from build123d import *

# Parameters (mm, degrees)
FILLET1_R   = 0.2
HEX_2_DEPTH = 1.56


with BuildPart() as part:
    # BodySke → BaseBody (revolve)
    with BuildSketch(Plane.XY):
        with BuildLine():
            Line((12.75, 0), (12.75, 2.055))
            Line((12.75, 2.055), (12.305, 2.5))
            Line((12.305, 2.5), (2.75, 2.5))
            Line((2.75, 2.5), (2.75, 4.75))
            Line((2.75, 4.75), (2.37, 4.75))
            ThreePointArc((2.37, 4.75), (0.992680215, 3.754414901), (0, 2.375))
            Line((0, 2.375), (0, 0))
            Line((0, 0), (12.75, 0))
        make_face()
    revolve(axis=Axis((0, 0, 0), (1, 0, 0)))

    # Fillet1
    fillet1_edges = [part.edges().sort_by_distance(p)[0] for p in [
        (2.75, -2.5, 0),
    ]]
    fillet(fillet1_edges, radius=FILLET1_R)

    # Sketch2 → PreBroach (revolve, cut)
    with BuildSketch(Plane.XY):
        Polygon((0, 1.5), (1.56, 1.5), (2.426025404, 0), (0, 0), align=None)
    revolve(axis=Axis((0, 0, 0), (1, 0, 0)), mode=Mode.SUBTRACT)

    # Sketch3 → Hex 2 (cut)
    with BuildSketch(Plane(origin=(0, 0, 0), x_dir=(0, 0, -1), z_dir=(1, 0, 0))):
        Polygon((-1.5, -0.866025404), (-1.5, 0.866025404), (0, 1.732050808), (1.5, 0.866025404), (1.5, -0.866025404), (0, -1.732050808), align=None)
    extrude(amount=HEX_2_DEPTH, mode=Mode.SUBTRACT)


solid = part.part
Check sheet for the modelled part. Datum: model origin and axes. Units: mm. A direction names the side the tool comes from. Give positions to 0.01 mm unless a question says otherwise; leave off trailing zeros. Loops run counter-clockwise (first coordinate to the right, second up) from the corner with the lowest first, then second, coordinate; pieces in that order, holes last. Notation, with made-up numbers: M -4.75,55 L 0.25,55 A10 ccw 0.25,62 Z; hole C 23,63.5 d9. An arc over 180 degrees is marked long. Answer as a JSON object with one key per item and string values. Group by question number.
Q1. Material ranges on line 1 along Z through (x, y) = (3.25, 2); line 2 along X through (y, z) = (2.75, -3.5); line 3 along X through (y, z) = (-4.5, -0.5), recorded low to high. Write a range as [from, to].
Q2. Cross-section at A-A on x = 1. Record the cut outline in (y, z).
Q3. Cross-section at C-C on z = -3.75. Record the cut outline in (x, y), then the cut area to 3 significant figures.
Q4. Go/stop test with flat-tipped pins: P1, Ø1.5, axis at x = 8, z = -1.5, coming from the -Y side; P2, Ø4, axis at y = 3, z = -3, coming from the +X side; P3, Ø3, axis at x = 9.5, z = -3, coming from the +Y side. Record where each tip stops, or that it passes through.
Q5. Cross-section at B-B on x = 11.25. Record the cut outline in (y, z).
Q6. Release check for a two-part mould opening along Y. For faces 1 (the flat face through (0.769, 1.305, -0.74)), 2 (the cylindrical face through (2.557, 2.192, -4.214)), 3 (the flat face through (0, 0, -2)), 4 (the flat face through (0.769, -1.293, -0.76)) record: released by +Y, released by -Y, zero draft, split by the parting line, or undercut.
Q7. Access from +Z, -Z, +X, -X, +Y, -Y to the whole of each face (thin tool, end or side, straight path). Record for faces 5 (the flat face through (2.75, -2.04, -2.04)), 6 (the flat face through (12.75, 0, 0)), 7 (the flat face through (0.769, 1.293, 0.76)).
Evaluation:
{
 "1": {"line 1": "z = [-1.5, 1.5]", "line 2": "x = [1.85, 2.75]", "line 3": "x = [1.97, 2.75]"},
 "2": {"outline": "C 0,0 d7.52; hole M -1.73,0 L -0.87,-1.5 L 0.87,-1.5 L 1.73,0 L 0.87,1.5 L -0.87,1.5 Z"},
 "3": {"outline": "M 2.37,-2.92 L 2.75,-2.92 L 2.75,2.92 L 2.37,2.92 A3.77 ccw Z", "area": "7.82 mm2"},
 "4": {"P1": "stops at y = -2.38", "P2": "stops at x = 12.56", "P3": "stops at y = 2"},
 "5": {"outline": "C 0,0 d5"},
 "6": {"face 1": "undercut", "face 2": "split by the parting line", "face 3": "zero draft", "face 4": "undercut"},
 "7": {"face 5": "+X", "face 6": "+Z, -Z, +X, +Y, -Y", "face 7": "-X"}
}
